For this review, take the finished solid that the model builds, in its own axes (mm). Coordinates: 2 decimals unless noted, no trailing zeros. Loops run counter-clockwise (first coordinate to the right, second up) from the corner with the lowest first, then second, coordinate; pieces in that order, holes last. Notation, with made-up numbers: (73.25, 30) - (95.25, 30) arc R34 cw to (95.25, 69) - close; hole circle Ø3 at (28.25, 75). An arc over 180 degrees is marked (long way). One line per item, written item: value. Start each with the question number.
1. Take a section at D-D, the plane x = 38. State the section outline as (y, z) points, and give its area (3 significant figures).
2. Insertion check: pin 1 (12 mm diameter, centred on x = 28.5, z = 23.5, fed in from -Y); pin 2 (1.2 mm diameter, centred on x = -11, y = 2, fed in from -Z); pin 3 (2 mm diameter, centred on y = 3, z = 0.5, fed in from -X); pin 4 (2 mm diameter, centred on y = 2, z = 2.5, fed in from +X). Each pin has a flat end and moves straight along its axis. Give the tip position at first contact, or say it passes through.
3. Take a section at B-B, the plane z = 2. Count the separate pieces of the cut face and the enclosed holes in it, and give its area (3 significant figures).
4. Take a section at A-A, the plane y = 1.3. State the section outline as (x, z) points.
5. To check wall thickness, follow line 1 (Z direction, x = 25, y = 2.8); line 2 (X direction, y = 2.5, z = 23); line 3 (X direction, y = 2.55, z = 1). State the ranges of each line that lie inside material, in increasing order. Write a range as from..to.
6. Take a section at C-C, the plane z = 11.5. State the section outline as (x, y) points, and give its area (3 significant figures).
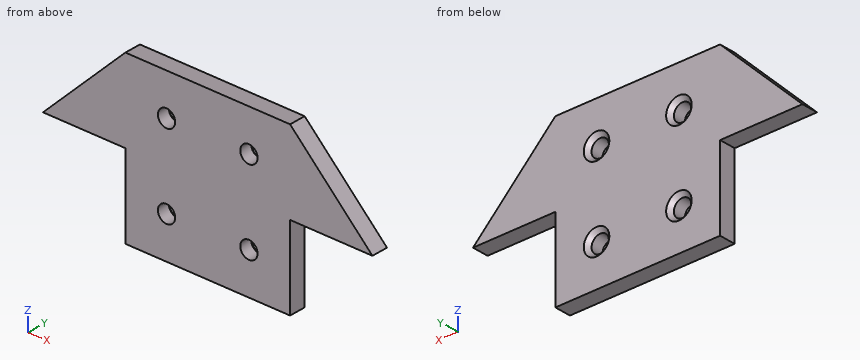
```python
from build123d import *

# Parameters (mm, degrees)
BOSS_EXTRUDE1_DEPTH = 4
SKETCH2_R           = 2.1
CUT_EXTRUDE1_DEPTH  = 4
CHAMFER1_SIZE       = 1


with BuildPart() as part:
    # Sketch1 → Boss-Extrude1 (new body)
    with BuildSketch(Plane(origin=(0, 0, 0), x_dir=(1, 0, 0), z_dir=(0, 1, 0))):
        Polygon((-4.540045767, -33.235697941), (35.459954233, -33.235697941), (55.459954233, -13.235697941), (35.459954233, -13.235697941), (35.459954233, 6.764302059), (-4.540045767, 6.764302059), (-4.540045767, -13.235697941), (-24.540045767, -13.235697941), align=None)
    extrude(amount=BOSS_EXTRUDE1_DEPTH)

    # Sketch2 → Cut-Extrude1 (cut)
    with BuildSketch(Plane(origin=(0, 4, 0), x_dir=(1, 0, 0), z_dir=(0, 1, 0))):
        with Locations((5.459954233, -23.235697941)):
            Circle(SKETCH2_R)
        with Locations((25.459954233, -23.235697941)):
            Circle(SKETCH2_R)
        with Locations((25.459954233, -3.235697941)):
            Circle(SKETCH2_R)
        with Locations((5.459954233, -3.235697941)):
            Circle(SKETCH2_R)
    extrude(amount=-CUT_EXTRUDE1_DEPTH, mode=Mode.SUBTRACT)

    # Chamfer1
    chamfer1_edges = [part.edges().sort_by_distance(p)[0] for p in [
        (3.359954233, 4, 3.235697941),
        (23.359954233, 4, 3.235697941),
        (23.359954233, 4, 23.235697941),
        (3.359954233, 4, 23.235697941),
    ]]
    chamfer(chamfer1_edges, length=CHAMFER1_SIZE)


solid = part.part
```
Solutions:
1. outline: (0, 13.24) - (4, 13.24) - (4, 30.7) - (0, 30.7) - close
1. area: 69.8 mm2
2. pin 1: y = 0
2. pin 2: z = 13.24
2. pin 3: x = -4.54
2. pin 4: x = 35.46
3. separate pieces: 3
3. enclosed holes: 0
3. area: 130 mm2
4. outline: (-24.54, 13.24) - (-4.54, 13.24) - (-4.54, -6.76) - (35.46, -6.76) - (35.46, 13.24) - (55.46, 13.24) - (35.46, 33.24) - (-4.54, 33.24) - close; hole circle Ø4.2 at (5.46, 3.24); hole circle Ø4.2 at (5.46, 23.24); hole circle Ø4.2 at (25.46, 3.24); hole circle Ø4.2 at (25.46, 23.24)
5. line 1: -6.76..1.19, 5.28..21.19, 25.28..33.24
5. line 2: -14.78..3.37, 7.55..23.37, 27.55..45.7
5. line 3: -4.54..35.46
6. outline: (-4.54, 0) - (35.46, 0) - (35.46, 4) - (-4.54, 4) - close
6. area: 160 mm2
